Can you work these out from the model? Positions are in its coordinate system, mm. A direction names the side the tool comes from. Give positions to 0.01 mm unless a question says otherwise; leave off trailing zeros. Order: outer loops, then holes, each group sorted by start corner. A loop starts at its lowest first (then second) coordinate and runs counter-clockwise, first axis right, second up. Notation, with made-up numbers: (48.25, -35.5) - (90.25, -35.5) arc R21 cw to (90.25, -17.5) - close; hole circle Ø6 at (76, 71.25). An arc over 180 degrees is marked (long way). Use one line per item in the form item = value. Start each with the question number.
1) Please list where these lines run through material, in increasing order: probe 1 along Y at (x, z) = (1.5, 108.5); probe 2 along Z at (x, y) = (-0.5, 50.5); probe 3 along Y at (x, z) = (0, 129.5).
2) We'd pull the mould along Y, two halves only. Please class faces 3 (the flat face through (0, 63.246, 111)), 4 (the flat face through (0, -53, 97.057)), 5 (the flat face through (0, -1, 89.437)), 6 (the flat face through (0, 53, 97.057)): released by +Y, released by -Y, zero draft, split by the parting line, or undercut.
3) Suppose I cut it at C-C, the plane y = 51. Write out the boundary of the cut face in (x, z).
4) Suppose I cut it at B-B, the plane x = 1.5. Write out the boundary of the cut face in (y, z).
5) Which directions (+Z, -Z, +X, -X, +Y, -Y) give clear straight access to the entire face, cutting with the end or side of a thin tool? Please do faces 1 (the flat face through (0, -49.53, 111)), 2 (the flat face through (0, -63.246, 111)).
6) Suppose I cut it at A-A, the plane z = 116.5. Write out the boundary of the cut face in (x, y), and give its area (3 significant figures).
```python
from build123d import *

# Parameters (mm, degrees)
SKETCH1_W           = 43.18
SKETCH1_H           = 126.492
SKETCH1_W_2         = 27.94
SKETCH1_H_2         = 6.096
BOSS_EXTRUDE1_DEPTH = 3.048
CHAMFER1_SIZE       = 3.81


with BuildPart() as part:
    # Sketch1 → Boss-Extrude1 (new body, symmetric)
    with BuildSketch(Plane(origin=(0, 0, 0), x_dir=(0, 0, -1), z_dir=(1, 0, 0))):
        with Locations((-111.027292876, 0)):
            Rectangle(SKETCH1_W, SKETCH1_H)
        with Locations((-111.027292876, 52.578)):
            Rectangle(SKETCH1_W_2, SKETCH1_H_2, mode=Mode.SUBTRACT)
        with Locations((-111.027292876, -52.578)):
            Rectangle(SKETCH1_W_2, SKETCH1_H_2, mode=Mode.SUBTRACT)
    extrude(amount=BOSS_EXTRUDE1_DEPTH, both=True)

    # Chamfer1
    chamfer1_edges = [part.edges().sort_by_distance(p)[0] for p in [
        (0, -63.246, 89.437292876),
        (0, -63.246, 132.617292876),
        (0, 63.246, 132.617292876),
        (0, 63.246, 89.437292876),
    ]]
    chamfer(chamfer1_edges, length=CHAMFER1_SIZE)


solid = part.part
```
Result sheet:
q1.probe_1 = -63.25 to -55.63, -49.53 to 49.53, 55.63 to 63.25
q1.probe_2 = 89.44 to 97.06, 125 to 132.62
q1.probe_3 = -62.55 to 62.55
q2.face_3 = released by +Y
q2.face_4 = undercut
q2.face_5 = zero draft
q2.face_6 = undercut
q3.outline = (-3.05, 89.44) - (3.05, 89.44) - (3.05, 97.06) - (-3.05, 97.06) - close; (-3.05, 125) - (3.05, 125) - (3.05, 132.62) - (-3.05, 132.62) - close
q4.outline = (-63.25, 93.25) - (-59.44, 89.44) - (59.44, 89.44) - (63.25, 93.25) - (63.25, 128.81) - (59.44, 132.62) - (-59.44, 132.62) - (-63.25, 128.81) - close; hole (-55.63, 97.06) - (-49.53, 97.06) - (-49.53, 125) - (-55.63, 125) - close; hole (49.53, 97.06) - (55.63, 97.06) - (55.63, 125) - (49.53, 125) - close
q5.face_1 = +X, -X
q5.face_2 = +Z, -Z, +X, -X, -Y
q6.outline = (-3.05, -63.25) - (3.05, -63.25) - (3.05, -55.63) - (-3.05, -55.63) - close; (-3.05, -49.53) - (3.05, -49.53) - (3.05, 49.53) - (-3.05, 49.53) - close; (-3.05, 55.63) - (3.05, 55.63) - (3.05, 63.25) - (-3.05, 63.25) - close
q6.area = 697 mm²
